The model under review builds one solid part; all positions refer to its coordinate system, in mm. A direction names the side the tool comes from. Coordinates: 2 decimals unless noted, no trailing zeros. Order: outer loops, then holes, each group sorted by start corner. A loop starts at its lowest first (then second) coordinate and runs counter-clockwise, first axis right, second up. Notation, with made-up numbers: (13.5, -4.5) -> (30.5, -4.5) arc R12 ccw to (30.5, 1.5) -> close; hole circle Ø6 at (-7, -7). An arc over 180 degrees is marked (long way). Put each result on its own line as item: value.
from build123d import *

# Parameters (mm, degrees)
SKETCH_1_W          = 26.5
SKETCH_1_H          = 33
SKETCH_1_R          = 4.9
SKETCH_1_R_2        = 1.65
EXTRUDE_1_DEPTH     = 3.3
SKETCH_2_W          = 26.5
SKETCH_2_H          = 3.3
EXTRUDE_2_DEPTH     = 34
CUT_EXTRUDE_3_DEPTH = 34
SKETCH_4_R          = 4
SKETCH_4_R_2        = 1.5
CUT_EXTRUDE_4_DEPTH = 34


with BuildPart() as part:
    # 草图1 → 凸台-拉伸1 (new body)
    with BuildSketch(Plane(origin=(0, 0, 0), x_dir=(1, 0, 0), z_dir=(0, 1, 0))):
        with Locations((13.25, 16.5)):
            Rectangle(SKETCH_1_W, SKETCH_1_H)
        with Locations(Location((12.525580031, 17.8, 0), (0, 0, 270))):
            Circle(SKETCH_1_R, mode=Mode.SUBTRACT)
        with Locations(Location((4.525580031, 24.85, 0), (0, 0, 270))):
            Circle(SKETCH_1_R_2, mode=Mode.SUBTRACT)
        with Locations(Location((20.525580031, 24.85, 0), (0, 0, 90))):
            Circle(SKETCH_1_R_2, mode=Mode.SUBTRACT)
        with Locations(Location((4.525580031, 10.85, 0), (0, 0, 270))):
            Circle(SKETCH_1_R_2, mode=Mode.SUBTRACT)
        with Locations(Location((20.525580031, 10.85, 0), (0, 0, 270))):
            Circle(SKETCH_1_R_2, mode=Mode.SUBTRACT)
    extrude(amount=EXTRUDE_1_DEPTH)

    # 草图2 → 凸台-拉伸2 (add)
    with BuildSketch(Plane(origin=(0, 3.3, 0), x_dir=(1, 0, 0), z_dir=(0, 1, 0))):
        with Locations((13.25, 1.65)):
            Rectangle(SKETCH_2_W, SKETCH_2_H)
    extrude(amount=EXTRUDE_2_DEPTH)

    # 草图3 → 切除-拉伸3 (cut)
    with BuildSketch(Plane(origin=(0, 0, -3.3), x_dir=(-1, 0, 0), z_dir=(0, 0, -1))):
        with BuildLine():
            Line((-26.5, 37.3), (-26.5, 24.05))
            ThreePointArc((-26.5, 24.05), (-22.619164851, 33.419164851), (-13.25, 37.3))
            Line((-13.25, 37.3), (-26.5, 37.3))
        make_face()
        with BuildLine():
            ThreePointArc((-13.25, 37.3), (-3.880835149, 33.419164851), (0, 24.05))
            Line((0, 24.05), (0, 37.3))
            Line((0, 37.3), (-13.25, 37.3))
        make_face()
    extrude(amount=-CUT_EXTRUDE_3_DEPTH, mode=Mode.SUBTRACT)

    # 草图4 → 切除-拉伸4 (cut)
    with BuildSketch(Plane(origin=(0, 0, -3.3), x_dir=(-1, 0, 0), z_dir=(0, 0, -1))):
        with Locations((-13.25, 24.05)):
            Circle(SKETCH_4_R)
        with Locations((-4.75, 24.05)):
            Circle(SKETCH_4_R_2)
        with Locations((-21.75, 24.05)):
            Circle(SKETCH_4_R_2)
    extrude(amount=-CUT_EXTRUDE_4_DEPTH, mode=Mode.SUBTRACT)


solid = part.part
Item 1: Consider section D-D on x = 16. Write out the cut boundary in (y, z).
Answers below:
outline: (0, -33) -> (3.3, -33) -> (3.3, -21.26) -> (0, -21.26) -> close; (0, -14.34) -> (3.3, -14.34) -> (3.3, -3.3) -> (21.15, -3.3) -> (21.15, 0) -> (0, 0) -> close; (26.95, -3.3) -> (37.01, -3.3) -> (37.01, 0) -> (26.95, 0) -> close
Item 2: Consider section A-A on z = -10.85. Write out the cut boundary in (x, y), and give its area (3 significant figures).
Answers below:
outline: (0, 0) -> (2.88, 0) -> (2.88, 3.3) -> (0, 3.3) -> close; (6.18, 0) -> (18.88, 0) -> (18.88, 3.3) -> (6.18, 3.3) -> close; (22.18, 0) -> (26.5, 0) -> (26.5, 3.3) -> (22.18, 3.3) -> close
area: 65.7 mm^2
Item 3: For pin 1 Ø10 at (x, y) = (16, 23.5) entering from -Z; pin 2 Ø12 at (x, z) = (3, -27.5) entering from +Y; pin 3 Ø10 at (x, z) = (20.5, -27) entering from -Y, all flat-tipped, find the tip position at first contact; note any pin that passes through.
Answers below:
pin 1: z = -3.3
pin 2: y = 3.3
pin 3: y = 0
Item 4: Consider section B-B on x = 5.25. Write out the cut boundary in (y, z).
Answers below:
outline: (0, -33) -> (3.3, -33) -> (3.3, -26.33) -> (0, -26.33) -> close; (0, -23.37) -> (3.3, -23.37) -> (3.3, -12.33) -> (0, -12.33) -> close; (0, -9.37) -> (3.3, -9.37) -> (3.3, -3.3) -> (22.64, -3.3) -> (22.64, 0) -> (0, 0) -> close; (25.46, -3.3) -> (34.61, -3.3) -> (34.61, 0) -> (25.46, 0) -> close
Item 5: For line 1 (X direction, y = 1.9, z = -17.8); line 2 (Z direction, x = 17.25, y = 23.5); line 3 (Y direction, x = 17.75, z = -9), list the stretches that pass through material, from the lowest coordinate up. Write a range as from..to.
Answers below:
line 1: 0..7.63, 17.43..26.5
line 2: -3.3..0
line 3: 0..3.3
Item 6: Mouldability with a two-part tool opening along Y and no side actions: class faces 3 (the flat face through (16, 0, -13)), 4 (the flat face through (16, 3.3, -22)), 5 (the flat face through (0, 2, -10)), 6 (the cylindrical face through (5.075, 22.586, -1.673)) as +Y half, -Y half, draft (parallel to the pull), parting line (faces both ways), or undercut.
Answers below:
face 3: -Y half
face 4: +Y half
face 5: draft
face 6: undercut
Item 7: Consider section C-C on z = -22. Write out the cut boundary in (x, y).
Answers below:
outline: (0, 0) -> (10, 0) -> (10, 3.3) -> (0, 3.3) -> close; (15.05, 0) -> (26.5, 0) -> (26.5, 3.3) -> (15.05, 3.3) -> close
Item 8: For faces 1 (the flat face through (13, 16, -3.3)), 2 (the flat face through (13, 2, -33)), list the 3-axis set-ups (+Z, -Z, +X, -X, +Y, -Y) from which the entire face can be reached by the end or side of a thin tool; tool diameter is ignored.
Answers below:
face 1: -Z, +X, -X, +Y
face 2: -Z, +X, -X, +Y, -Y
